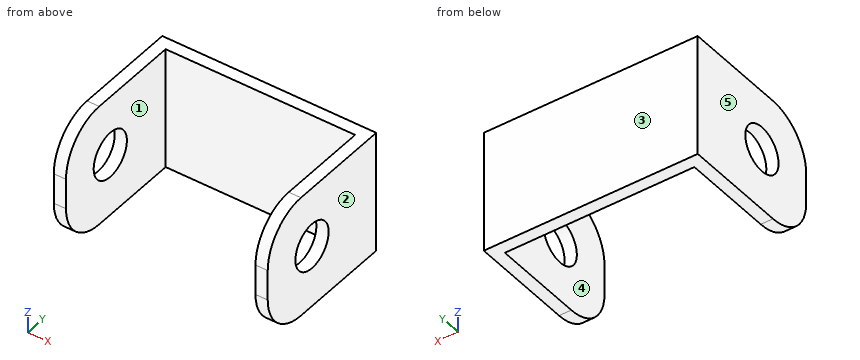
```python
from build123d import *

# Parameters (mm, degrees)
SKETCH1_W           = 35.56
SKETCH1_H           = 20.32
BOSS_EXTRUDE1_DEPTH = 2.032
SKETCH2_W           = 2.032
SKETCH2_H           = 20.32
BOSS_EXTRUDE2_DEPTH = 22.86
FILLET1_R           = 7.62
SKETCH3_R           = 3.81
CUT_EXTRUDE1_DEPTH  = 49.022


with BuildPart() as part:
    # Sketch1 → Boss-Extrude1 (new body)
    with BuildSketch(Plane(origin=(0, 0, 0), x_dir=(1, 0, 0), z_dir=(0, 1, 0))):
        with Locations((3.501518098, 0.190585347)):
            Rectangle(SKETCH1_W, SKETCH1_H)
    extrude(amount=BOSS_EXTRUDE1_DEPTH)

    # Sketch2 → Boss-Extrude2 (add)
    with BuildSketch(Plane.XZ):
        with Locations((-13.262481902, -0.190585347)):
            Rectangle(SKETCH2_W, SKETCH2_H)
        with Locations((20.265518098, -0.190585347)):
            Rectangle(SKETCH2_W, SKETCH2_H)
    extrude(amount=BOSS_EXTRUDE2_DEPTH)

    # Fillet1
    fillet1_edges = [part.edges().sort_by_distance(p)[0] for p in [
        (-13.262481902, -22.86, -10.350585347),
        (-13.262481902, -22.86, 9.969414653),
        (20.265518098, -22.86, 9.969414653),
        (20.265518098, -22.86, -10.350585347),
    ]]
    fillet(fillet1_edges, radius=FILLET1_R)

    # Sketch3 → Cut-Extrude1 (cut)
    with BuildSketch(Plane(origin=(21.281518098, 0, 0), x_dir=(0, 0, -1), z_dir=(1, 0, 0))):
        with Locations((0, -12.7)):
            Circle(SKETCH3_R)
    extrude(amount=-CUT_EXTRUDE1_DEPTH, mode=Mode.SUBTRACT)


solid = part.part
```
Geometry: final body of the model. Coordinates: model frame, mm. Face numbers are marked on the shaded views. A direction names the side the tool comes from. Coordinates: 2 decimals unless noted, no trailing zeros. Order: outer loops, then holes, each group sorted by start corner. A loop starts at its lowest first (then second) coordinate and runs counter-clockwise, first axis right, second up.
Item 1: Section query A-A (z = 0). Output: boundary loops of the cut face in (x, y).
Answer:
outline: (-14.28, -22.86) - (-12.25, -22.86) - (-12.25, -16.51) - (-14.28, -16.51) - close; (-14.28, -8.89) - (-12.25, -8.89) - (-12.25, 0) - (19.25, 0) - (19.25, -8.89) - (21.28, -8.89) - (21.28, 2.03) - (-14.28, 2.03) - close; (19.25, -22.86) - (21.28, -22.86) - (21.28, -16.51) - (19.25, -16.51) - close
Item 2: Material intervals for line 1 along X through (y, z) = (-4.75, -8.75); line 2 along Y through (x, z) = (20.25, 0); line 3 along Y through (x, z) = (16, -6.5), sorted ascending.
Answer:
line 1: x = -14.28 to -12.25, 19.25 to 21.28
line 2: y = -22.86 to -16.51, -8.89 to 2.03
line 3: y = 0 to 2.03
Item 3: Draft query along X for the marked faces 1, 2 and 3. Return one class per face: released by +X, released by -X, zero draft, split by the parting line, or undercut.
Answer:
face 1: undercut
face 2: released by +X
face 3: zero draft
Item 4: Section query D-D (z = -4.5). Output: boundary loops of the cut face in (x, y).
Answer:
outline: (-14.28, -22.65) - (-12.25, -22.65) - (-12.25, 0) - (19.25, 0) - (19.25, -22.65) - (21.28, -22.65) - (21.28, 2.03) - (-14.28, 2.03) - close
Item 5: Contact query for flat-ended pins moving along their axis: P1, Ø6, axis at x = 5.5, z = -6.5, coming from the -Y side; P2, Ø7, axis at y = -12.7, z = 0, coming from the -X side; P3, Ø10, axis at y = -12.7, z = 0, coming from the -X side. Output: stop coordinate, or through.
Answer:
P1: stops at y = 0
P2: passes through
P3: stops at x = -14.28
Item 6: Section query C-C (y = -12.7). Output: boundary loops of the cut face in (x, z).
Answer:
outline: (-14.28, -10.35) - (-12.25, -10.35) - (-12.25, -3.81) - (-14.28, -3.81) - close; (-14.28, 3.81) - (-12.25, 3.81) - (-12.25, 9.97) - (-14.28, 9.97) - close; (19.25, -10.35) - (21.28, -10.35) - (21.28, -3.81) - (19.25, -3.81) - close; (19.25, 3.81) - (21.28, 3.81) - (21.28, 9.97) - (19.25, 9.97) - close
Item 7: Access query for the marked faces 4 and 5. Directions: +Z, -Z, +X, -X, +Y, -Y. A direction counts if a zero-diameter tool reaches every point of the face in a straight line with its end or side. Return the directions, or none.
Answer:
face 4: +Z, -Z, -Y
face 5: +Z, -Z, -X, +Y, -Y
Item 8: Section query B-B (y = -3). Output: boundary loops of the cut face in (x, z).
Answer:
outline: (-14.28, -10.35) - (-12.25, -10.35) - (-12.25, 9.97) - (-14.28, 9.97) - close; (19.25, -10.35) - (21.28, -10.35) - (21.28, 9.97) - (19.25, 9.97) - close
